Design review of the part built by this model. Coordinates are the model's own, in mm. A direction names the side the tool comes from. Coordinates: 2 decimals unless noted, no trailing zeros. Order: outer loops, then holes, each group sorted by start corner. A loop starts at its lowest first (then second) coordinate and runs counter-clockwise, first axis right, second up. Notation, with made-up numbers: M 44.5,46 L 59.5,46 A20 ccw 59.5,64 Z; hole C 77,60.5 d2. An arc over 180 degrees is marked long. Answer as a JSON object with one key per item and string values.
from build123d import *

# Parameters (mm, degrees)
SKETCH_7_W                  = 400
SKETCH_7_H                  = 330
EXTRUDE_6_DEPTH             = 16
SKETCH_8_R                  = 13
CUT_EXTRUDE_2_DEPTH         = 519.802467226
PATTERN_LINEAR_1_COUNT      = 2
PATTERN_LINEAR_1_PITCH      = 300
PATTERN_LINEAR_1_COUNT_DIR2 = 4
PATTERN_LINEAR_1_PITCH_DIR2 = 80
SKETCH_9_W                  = 382
SKETCH_9_H                  = 16
EXTRUDE_7_DEPTH             = 261
CUT_EXTRUDE_3_DEPTH         = 497.718229986
EXTRUDE_8_DEPTH             = 192
EXTRUDE_9_DEPTH             = 192
SKETCH_13_W                 = 330
SKETCH_13_H                 = 400
EXTRUDE_10_DEPTH            = 16
SKETCH_14_R                 = 13
CUT_EXTRUDE_4_DEPTH         = 16
PATTERN_LINEAR_2_COUNT      = 4
PATTERN_LINEAR_2_PITCH      = 80
PATTERN_LINEAR_2_COUNT_DIR2 = 2
PATTERN_LINEAR_2_PITCH_DIR2 = 300


with BuildPart() as part:
    # 草图7 → 凸台-拉伸6 (new body)
    with BuildSketch(Plane(origin=(0, 0, 0), x_dir=(0, -1, 0), z_dir=(1, 0, 0))):
        with Locations((200, 165)):
            Rectangle(SKETCH_7_W, SKETCH_7_H)
    extrude(amount=EXTRUDE_6_DEPTH)

    # 草图8 → 切除-拉伸2 (cut, through all)
    with BuildSketch(Plane(origin=(16, 0, 0), x_dir=(0, -1, 0), z_dir=(1, 0, 0))):
        with Locations(Location((50, 45, 0), (0, 0, 180))):
            Circle(SKETCH_8_R)
    cut_extrude_2 = extrude(amount=-CUT_EXTRUDE_2_DEPTH, mode=Mode.SUBTRACT)

    # 阵列(线性)1: Cut-Extrude 2 2 × 4
    with Locations(*[(0, -i * PATTERN_LINEAR_1_PITCH, -j * PATTERN_LINEAR_1_PITCH_DIR2) for i in range(PATTERN_LINEAR_1_COUNT) for j in range(PATTERN_LINEAR_1_COUNT_DIR2) if (i, j) != (0, 0)]):
        add(cut_extrude_2, mode=Mode.SUBTRACT)

    # 草图9 → 凸台-拉伸7 (add)
    with BuildSketch(Plane(origin=(16, 0, 0), x_dir=(0, 0, -1), z_dir=(1, 0, 0))):
        with Locations((165, -200)):
            Rectangle(SKETCH_9_W, SKETCH_9_H)
    extrude(amount=EXTRUDE_7_DEPTH)

    # 草图10 → 切除-拉伸3 (cut, through all)
    with BuildSketch(Plane(origin=(0, -208, 0), x_dir=(-1, 0, 0), z_dir=(0, -1, 0))):
        Polygon((-16, -26), (-16, 0), (-277, -26), align=None)
        Polygon((-16, 330), (-277, 304), (-277, 356), (-16, 356), align=None)
    extrude(amount=-CUT_EXTRUDE_3_DEPTH, mode=Mode.SUBTRACT)

    # 草图11 → 凸台-拉伸8 (add)
    with BuildSketch(Plane.XZ.offset(208)):
        Polygon((16, -79.579291616), (277, -53.579291616), (277, -63.62878672), (16, -89.62878672), align=None)
        Polygon((16, -170.024747552), (277, -144.024747552), (277, -133.975252448), (16, -159.975252448), align=None)
        Polygon((16, -240.37121328), (277, -214.37121328), (277, -224.420708384), (16, -250.420708384), align=None)
    extrude(amount=EXTRUDE_8_DEPTH)

    # 草图12 → 凸台-拉伸9 (add)
    with BuildSketch(Plane(origin=(0, -192, 0), x_dir=(1, 0, 0), z_dir=(0, 1, 0))):
        Polygon((16, 79.579291616), (16, 89.62878672), (277, 63.62878672), (277, 53.579291616), align=None)
        Polygon((16, 159.975252448), (16, 170.024747552), (277, 144.024747552), (277, 133.975252448), align=None)
        Polygon((16, 240.37121328), (16, 250.420708384), (277, 224.420708384), (277, 214.37121328), align=None)
    extrude(amount=EXTRUDE_9_DEPTH)

    # 草图13 → 凸台-拉伸10 (add)
    with BuildSketch(Plane(origin=(277, 0, 0), x_dir=(0, 0, -1), z_dir=(1, 0, 0))):
        with Locations((139, -200)):
            Rectangle(SKETCH_13_W, SKETCH_13_H)
    extrude(amount=EXTRUDE_10_DEPTH)

    # 草图14 → 切除-拉伸4 (cut)
    with BuildSketch(Plane(origin=(293, 0, 0), x_dir=(0, 0, -1), z_dir=(1, 0, 0))):
        with Locations((19, -350)):
            Circle(SKETCH_14_R)
    cut_extrude_4 = extrude(amount=-CUT_EXTRUDE_4_DEPTH, mode=Mode.SUBTRACT)

    # 阵列(线性)2: Cut-Extrude 4 4 × 2
    with Locations(*[(0, j * PATTERN_LINEAR_2_PITCH_DIR2, -i * PATTERN_LINEAR_2_PITCH) for i in range(PATTERN_LINEAR_2_COUNT) for j in range(PATTERN_LINEAR_2_COUNT_DIR2) if (i, j) != (0, 0)]):
        add(cut_extrude_4, mode=Mode.SUBTRACT)


solid = part.part
1) Tool access review of faces 4 (the flat face through (145, -208, -26)), 5 (the cylindrical face through (285.11, -362.69, -96.18)), 6 (the flat face through (144.673, -302.656, -157.207)), 7 (the flat face through (277, -303, -264)): name each direction out of +Z, -Z, +X, -X, +Y, -Y from which nothing blocks a thin tool from reaching the whole face with its end or side.
Taken from the geometry:
{"face 4": "+Z, -Y", "face 5": "+X", "face 6": "-Y", "face 7": "-Z, -Y"}
2) To check wall thickness, follow L1, parallel to Y at x = 285.25, z = -179; L2, parallel to Z at x = 6.75, y = -50; L3, parallel to Z at x = 201, y = -56.5. State the ranges of each line that lie inside material, in increasing order.
Taken from the geometry:
{"L1": "y = -400 to -363, -337 to -63, -37 to 0", "L2": "z = -330 to -298, -272 to -218, -192 to -138, -112 to -58, -32 to 0", "L3": "z = -231.99 to -221.94, -151.6 to -141.55, -71.2 to -61.15"}
3) Add section A-A (y = -310.5). State the section outline as (x, z) points, and give its area (3 significant figures).
Taken from the geometry:
{"outline": "M 0,-330 L 16,-330 L 16,-250.42 L 277,-224.42 L 277,-304 L 293,-304 L 293,26 L 277,26 L 277,-53.58 L 16,-79.58 L 16,0 L 0,0 Z; hole M 16,-240.37 L 277,-214.37 L 277,-144.02 L 16,-170.02 Z; hole M 16,-159.98 L 277,-133.98 L 277,-63.63 L 16,-89.63 Z", "area": "18,400 mm2"}
4) Add section D-D (z = -22.5). State the section outline as (x, y) points, and give its area (3 significant figures).
Taken from the geometry:
{"outline": "M 0,-400 L 16,-400 L 16,-208 L 277,-208 L 277,-337.48 L 293,-337.48 L 293,-62.52 L 277,-62.52 L 277,-192 L 16,-192 L 16,0 L 0,0 Z; M 277,-400 L 293,-400 L 293,-362.52 L 277,-362.52 Z; M 277,-37.48 L 293,-37.48 L 293,0 L 277,0 Z", "area": "16,200 mm2"}
5) Add section B-B (z = -205). State the section outline as (x, y) points, and give its area (3 significant figures).
Taken from the geometry:
{"outline": "M 0,-400 L 16,-400 L 16,-363 L 0,-363 Z; M 0,-337 L 16,-337 L 16,-208 L 277,-208 L 277,-400 L 293,-400 L 293,0 L 277,0 L 277,-192 L 16,-192 L 16,-63 L 0,-63 Z; M 0,-37 L 16,-37 L 16,0 L 0,0 Z", "area": "16,100 mm2"}
6) Add section C-C (x = 88). State the section outline as (y, z) points.
Taken from the geometry:
{"outline": "M -400,-243.25 L -208,-243.25 L -208,-322.83 L -192,-322.83 L -192,-243.25 L 0,-243.25 L 0,-233.2 L -192,-233.2 L -192,-162.85 L 0,-162.85 L 0,-152.8 L -192,-152.8 L -192,-82.46 L 0,-82.46 L 0,-72.41 L -192,-72.41 L -192,7.17 L -208,7.17 L -208,-72.41 L -400,-72.41 L -400,-82.46 L -208,-82.46 L -208,-152.8 L -400,-152.8 L -400,-162.85 L -208,-162.85 L -208,-233.2 L -400,-233.2 Z"}
7) Mouldability with a two-part tool opening along Y and no side actions: class faces 1 (the flat face through (16, -95, -125)), 2 (the flat face through (145, -208, -192)), 3 (the cylindrical face through (8.112, -360.316, -212.91)) as released by +Y, released by -Y, zero draft, split by the parting line, or undercut.
Taken from the geometry:
{"face 1": "zero draft", "face 2": "released by -Y", "face 3": "undercut"}
8) Insertion check: pin 1 Ø3 at (x, y) = (51.5, -344) entering from -Z; pin 2 Ø1 at (x, y) = (124, -318) entering from -Z; pin 3 Ø10 at (x, y) = (120.5, -196) entering from +Z. Each pin has a flat end and moves straight along its axis. Give the tip position at first contact, or say it passes through.
Taken from the geometry:
{"pin 1": "stops at z = -247.03", "pin 2": "stops at z = -239.71", "pin 3": "stops at z = 10.91"}
